```python
from build123d import *

# Parameters (mm, degrees)
F0_W     = 1060
F0_H     = 600
F1_DEPTH = 4
F2_W     = 1060
F2_H     = 600
F3_DEPTH = 101.6
F4_T     = -50.8


with BuildPart() as f1:
    # F0 (on Top) → F1 (new body)
    with BuildSketch(Plane.XY):
        with Locations((530, -300)):
            Rectangle(F0_W, F0_H)
    extrude(amount=F1_DEPTH)

    # F2 (on face) → F3 (join)
    with BuildSketch(Plane.XY.offset(4)):
        with Locations((530, -300)):
            Rectangle(F2_W, F2_H)
    extrude(amount=F3_DEPTH)

    # F4
    f4_openings = [f1.faces().sort_by_distance(p)[0] for p in [
        (530, -300, 105.6),
    ]]
    offset(amount=F4_T, openings=f4_openings)


solid = f1.part
```
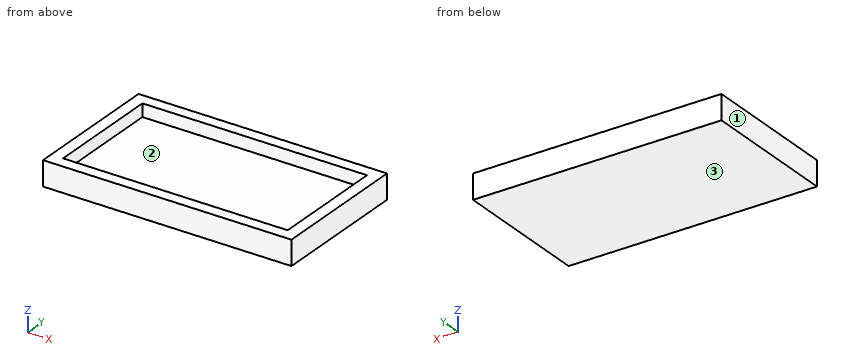
Geometry check sheet. Reference: the model listing, model coordinates, mm. Face numbers are marked on the shaded views. Coordinates: 2 decimals unless noted, no trailing zeros. Order: outer loops, then holes, each group sorted by start corner. A loop starts at its lowest first (then second) coordinate and runs counter-clockwise, first axis right, second up. Notation, with made-up numbers: M 7,38 L 19,38 A22 ccw 19,46 Z; hole C 60,13.5 d5. An arc over 180 degrees is marked long. Answer as a JSON object with one key per item and string values.
Q1. Cross-section at A-A on z = 89.5. Record the cut outline in (x, y), and give its area (3 significant figures).
Results are:
{"outline": "M 0,-600 L 1060,-600 L 1060,0 L 0,0 Z; hole M 50.8,-549.2 L 1009.2,-549.2 L 1009.2,-50.8 L 50.8,-50.8 Z", "area": "158,000 mm²"}
Q2. Release check for a two-part mould opening along X. For the marked faces 1, 2 and 3 record: released by +X, released by -X, zero draft, split by the parting line, or undercut.
Results are:
{"face 1": "released by -X", "face 2": "undercut", "face 3": "zero draft"}
Q3. Cross-section at B-B on x = 772. Record the cut outline in (y, z), and give its area (3 significant figures).
Results are:
{"outline": "M -600,0 L 0,0 L 0,105.6 L -50.8,105.6 L -50.8,50.8 L -549.2,50.8 L -549.2,105.6 L -600,105.6 Z", "area": "36,000 mm²"}
Q4. Scan lines: line 1 (X direction, y = -127.5, z = 62); line 2 (Y direction, x = 422, z = 71.5); line 3 (Z direction, x = 190.5, y = -55). Record each from-to range of solid material in increasing order.
Results are:
{"line 1": "x = 0 to 50.8, 1009.2 to 1060", "line 2": "y = -600 to -549.2, -50.8 to 0", "line 3": "z = 0 to 50.8"}
Q5. Cross-section at C-C on y = -121. Record the cut outline in (x, z), and give its area (3 significant figures).
Results are:
{"outline": "M 0,0 L 1060,0 L 1060,105.6 L 1009.2,105.6 L 1009.2,50.8 L 50.8,50.8 L 50.8,105.6 L 0,105.6 Z", "area": "59,400 mm²"}
Q6. Depth check by flat-ended pin: pin 1 Ø1.5 at (x, y) = (440.5, -500) entering from +Z. Enter the tip coordinate at first touch or a pass-through.
Results are:
{"pin 1": "stops at z = 50.8"}
